Could you check a few things on this model? Use its own coordinates, in mm. A direction names the side the tool comes from. Give positions to 0.01 mm unless a question says otherwise; leave off trailing zeros. Order: outer loops, then holes, each group sorted by start corner. A loop starts at its lowest first (then second) coordinate and runs counter-clockwise, first axis right, second up.
(1) If I drill on probe 1 along Y at (x, z) = (-11, 27.5); probe 2 along Y at (x, z) = (44.5, -6); probe 3 along Z at (x, y) = (27.5, -74), over which ranges is the centre line in solid material (lowest first)?
(2) Imagine slicing it at B-B, the plane y = -20. Write out the boundary of the cut face in (x, z).
(3) On a 3-axis mill with a long thin cutter (end or side, diameter ignored), from which of +Z, -Z, +X, -X, +Y, -Y can I reach the whole of each face in a straight line? I mean faces 1 (the flat face through (-18, -4, 22)), 2 (the flat face through (0, -17.5, -1)), 3 (the flat face through (10, -13, 30)). Say none if no direction works.
(4) Imagine slicing it at C-C, the plane x = -8.5. Write out the boundary of the cut face in (y, z), then the cut area to 3 significant figures.
(5) If we mould it in two halves opening along Y, with no side actions, what happens to faces 4 (the flat face through (-18, -21, 30)), 5 (the flat face through (-4, -25.5, 30)), 6 (the flat face through (0, -13, 25))? For each: released by +Y, released by -Y, zero draft, split by the parting line, or undercut.
(6) Imagine slicing it at A-A, the plane z = -5. Write out the boundary of the cut face in (x, y).
(7) Will these pins go through, and if not, where does the flat tip stop? pin 1 (20.5 mm diameter, centred on y = -16.5, z = 28.5, fed in from +X); pin 2 (0.6 mm diameter, centred on y = -8.5, z = -3, fed in from -X); pin 3 (0.6 mm diameter, centred on x = -2.5, y = -8, fed in from -Z).
(8) Imagine slicing it at D-D, the plane x = 18. Write out the boundary of the cut face in (y, z).
from build123d import *

# Parameters (mm, degrees)
BOSS_EXTRUDE1_DEPTH = 50
SKETCH2_W           = 7
SKETCH2_H           = 8
BOSS_EXTRUDE2_DEPTH = 50
SKETCH2_3_W         = 7
SKETCH2_3_H         = 8
BOSS_EXTRUDE3_DEPTH = 18
SKETCH3_W           = 10
SKETCH3_H           = 63
SKETCH3_W_2         = 7
SKETCH3_H_2         = 8
BOSS_EXTRUDE4_DEPTH = 82


with BuildPart() as part:
    # Sketch1 → Boss-Extrude1 (new body)
    with BuildSketch(Plane.XY):
        with BuildLine():
            Line((-1.5, -8), (-3.5, -8))
            ThreePointArc((-3.5, -8), (-2.5, -8.5), (-1.5, -8))
        make_face()
        Polygon((10, -25.5), (10, 0), (0, 0), (-18, 0), (-18, -8), (0, -8), (0, -17.5), (-18, -17.5), (-18, -25.5), align=None)
    extrude(amount=BOSS_EXTRUDE1_DEPTH)

    # Sketch2 → Boss-Extrude2 (add)
    with BuildSketch(Plane(origin=(0, 0, 0), x_dir=(0, 0, -1), z_dir=(1, 0, 0))):
        Polygon((7, 0), (0, 0), (0, -8), (1.5, -8), (3.5, -8), (7, -8), align=None)
        Polygon((0, -8), (0, 0), (-10, 0), (-10, -25.5), (0, -25.5), (0, -17.5), align=None)
        with Locations((3.5, -21.5)):
            Rectangle(SKETCH2_W, SKETCH2_H)
        with BuildLine():
            Line((3.5, -8), (1.5, -8))
            ThreePointArc((1.5, -8), (2.5, -8.5), (3.5, -8))
        make_face()
    extrude(amount=BOSS_EXTRUDE2_DEPTH)

    # Sketch2<3> → Boss-Extrude3 (add)
    with BuildSketch(Plane(origin=(0, 0, 0), x_dir=(0, 0, -1), z_dir=(1, 0, 0))):
        Polygon((7, 0), (0, 0), (0, -8), (1.5, -8), (3.5, -8), (7, -8), align=None)
        with Locations((3.5, -21.5)):
            Rectangle(SKETCH2_3_W, SKETCH2_3_H)
    extrude(amount=-BOSS_EXTRUDE3_DEPTH)

    # Sketch3 → Boss-Extrude4 (add)
    with BuildSketch(Plane(origin=(50, 0, 0), x_dir=(0, 0, -1), z_dir=(1, 0, 0))):
        Polygon((32.5, -17.5), (7, -17.5), (7, -25.5), (0, -25.5), (0, -88.5), (32.5, -88.5), align=None)
        with Locations((-5, -57)):
            Rectangle(SKETCH3_W, SKETCH3_H)
        with Locations((3.5, -21.5)):
            Rectangle(SKETCH3_W_2, SKETCH3_H_2)
        with Locations((-5, -21.5)):
            Rectangle(SKETCH3_W, SKETCH3_H_2)
    extrude(amount=-BOSS_EXTRUDE4_DEPTH)


solid = part.part
Answer block:
1. probe 1: y = -25.5 to -17.5, -8 to 0
1. probe 2: y = -88.5 to -17.5, -8 to 0
1. probe 3: z = -32.5 to 10
2. outline: (-32, -32.5) - (50, -32.5) - (50, 10) - (10, 10) - (10, 50) - (-18, 50) - (-18, 10) - (-32, 10) - close
3. face 1: +Z, -Z, -X, +Y
3. face 2: -Z, -X
3. face 3: +Z, +X, +Y, -Y
4. outline: (-88.5, -32.5) - (-17.5, -32.5) - (-17.5, 50) - (-25.5, 50) - (-25.5, 10) - (-88.5, 10) - close; (-8, -7) - (0, -7) - (0, 50) - (-8, 50) - close
4. area: 3,790 mm2
5. face 4: zero draft
5. face 5: released by -Y
5. face 6: undercut
6. outline: (-32, -88.5) - (50, -88.5) - (50, -17.5) - (-32, -17.5) - close; (-18, -8) - (50, -8) - (50, 0) - (-18, 0) - close
7. pin 1: stops at x = 10
7. pin 2: stops at x = 0
7. pin 3: stops at z = -7
8. outline: (-88.5, -32.5) - (-17.5, -32.5) - (-17.5, 0) - (-8, 0) - (-8, -1.5) arc R1.25 ccw to (-8, -3.5) - (-8, -7) - (0, -7) - (0, 10) - (-88.5, 10) - close
